Build history of the part. All positions in model axes, mm. A direction names the side the tool comes from. Round coordinates to 2 decimals unless told otherwise and drop trailing zeros. Write each loop counter-clockwise with the first axis right and the second up, starting at its lowest first coordinate (ties: lowest second). Pieces come first, ordered by that corner, then holes.
1) Saw through at A-A (y = 0). Write the cut outline in (x, z), plus the area to 3 significant figures.
2) Which spindle directions (+Z, -Z, +X, -X, +Y, -Y) get a long thin tool onto all of the face, cutting with end or side? Do faces 1 (the cylindrical face through (1.5, 0.07, -3.76)), 2 (the cylindrical face through (-2.38, -10.74, 11.83)), 3 (the cylindrical face through (-1.604, -7.224, 25.232)). Say none if no direction does.
3) Flat gauge pins, fed straight in: pin 1 (1.5 mm diameter, centred on x = -4, y = 8, fed in from +Z); pin 2 (5 mm diameter, centred on x = -1.5, z = 4, fed in from -Y); pin 3 (8 mm diameter, centred on x = 4, y = -8.5, fed in from -Z); pin 4 (4 mm diameter, centred on x = -6, z = -0.5, fed in from -Y). Where does each tip first touch, or does it go through?
4) Saw through at D-D (y = 4.75). Write the cut outline in (x, z).
5) Wall check: probe 1 along Z at (x, y) = (1.5, 1.5); probe 2 along Z at (x, y) = (7, -2); probe 3 along X at (y, z) = (7, 14). Give the ranges that are in metal, low to high.
6) Saw through at C-C (z = 9). Write the cut outline in (x, y), plus the area to 3 significant figures.
from build123d import *

# Parameters (mm, degrees)
SKETCH1_R      = 11
EXTRUDE1_DEPTH = 24
SKETCH2_R      = 7.4
EXTRUDE3_DEPTH = 2.5
SKETCH3_R      = 3.65
EXTRUDE4_DEPTH = 1.3
SKETCH4_R      = 1.5
EXTRUDE5_DEPTH = 5


with BuildPart() as part:
    # Sketch1 → Extrude1 (new body)
    with BuildSketch(Plane.XY):
        Circle(SKETCH1_R)
    extrude(amount=EXTRUDE1_DEPTH)

    # Sketch2 → Extrude3 (add)
    with BuildSketch(Plane.XY.offset(24)):
        Circle(SKETCH2_R)
    extrude(amount=EXTRUDE3_DEPTH)

    # Sketch3 → Extrude4 (add)
    with BuildSketch(Plane(origin=(0, 0, 0), x_dir=(-1, 0, 0), z_dir=(0, 0, -1))):
        Circle(SKETCH3_R)
    extrude(amount=EXTRUDE4_DEPTH)

    # Sketch4 → Extrude5 (add)
    with BuildSketch(Plane(origin=(0, 0, -1.3), x_dir=(-1, 0, 0), z_dir=(0, 0, -1))):
        Circle(SKETCH4_R)
    extrude(amount=EXTRUDE5_DEPTH)


solid = part.part
Evaluation:
1. outline: (-11, 0) - (-3.65, 0) - (-3.65, -1.3) - (-1.5, -1.3) - (-1.5, -6.3) - (1.5, -6.3) - (1.5, -1.3) - (3.65, -1.3) - (3.65, 0) - (11, 0) - (11, 24) - (7.4, 24) - (7.4, 26.5) - (-7.4, 26.5) - (-7.4, 24) - (-11, 24) - close
1. area: 589 mm2
2. face 1: -Z
2. face 2: +Z, -Z
2. face 3: +Z
3. pin 1: stops at z = 24
3. pin 2: stops at y = -11
3. pin 3: stops at z = 0
3. pin 4: stops at y = -10.22
4. outline: (-9.92, 0) - (9.92, 0) - (9.92, 24) - (5.67, 24) - (5.67, 26.5) - (-5.67, 26.5) - (-5.67, 24) - (-9.92, 24) - close
5. probe 1: z = -1.3 to 26.5
5. probe 2: z = 0 to 26.5
5. probe 3: x = -8.49 to 8.49
6. outline: circle Ø22 at (0, 0)
6. area: 380 mm2
